Autodesk Fusion 360 part; units mm, degrees
sketch "Sketch1" plane through (0, 0, 0) normal (0, 1, 0) x (1, 0, 0)
  line L0 (-70, 0) -> (50, 0)
  line L1 (-70, 0) -> (-70, 20)
  line L2 (-70, 20) -> (-80, 20)
  line L3 (-80, 20) -> (-80, -20)
  line L4 (-80, -20) -> (50.3493, -2.6201)
  line L5 (50, 0) -> (50.3493, -2.6201)
  line L6 (-70.3109, -13.2) -> (-62.1109, -13.2)
  line L7 (-62.1109, -13.2) -> (-62.1109, -5)
  line L8 (-62.1109, -5) -> (-70.3109, -5)
  line L9 (-70.3109, -5) -> (-70.3109, -13.2)
  line L10 (-9.6566, -8.2) -> (-4.4566, -8.2)
  line L11 (-4.4566, -8.2) -> (-4.4566, -3)
  line L12 (-4.4566, -3) -> (-9.6566, -3)
  line L13 (-9.6566, -3) -> (-9.6566, -8.2)
  dimension "d1" = 20
  dimension "d2" = 10
  dimension "d3" = 40
  dimension "d4" = 8.2
  dimension "d5" = 8.2
  dimension "d6" = 5
  dimension "d7" = 5.2
  dimension "d8" = 5.2
  dimension "d9" = 3
extrude "Extrude1" add sketch "Sketch1" along normal blind 8
fillet "Fillet1" radius 2 1 edges at (-70, 4, 0)
fillet "Fillet2" radius 6 1 edges at (-80, 4, -20)
fillet "Fillet3" radius 2.5 1 edges at (-70, 4, -20)
fillet "Fillet4" radius 2.5 1 edges at (-80, 4, 20)
fillet "Fillet5" radius 1.2 2 edges at (50.3493, 4, 2.6201) (50, 4, 0)
The listing builds one solid part. Answer for the finished solid, in the listing's coordinates (mm). A direction names the side the tool comes from. Give positions to 0.01 mm unless a question says otherwise; leave off trailing zeros. Loops run counter-clockwise (first coordinate to the right, second up) from the corner with the lowest first, then second, coordinate; pieces in that order, holes last. Notation, with made-up numbers: (-20, -14.75) - (-12, -14.75) arc R31 ccw to (-12, 17.25) - close; hole circle Ø6 at (-8.5, 5). An arc over 180 degrees is marked (long way). Write each question's results on one line, items separated by ' | '.
1. Which of the six approach directions +Z, -Z, +X, -X, +Y, -Y give full straight-line access (tool end or side, diameter ignored) to faces 1 (the face through (-34, 8, 4)), 2 (the face through (-4.457, 4, 6))?
Resolved:
face 1: +Z, -Z, +X, -X, +Y | face 2: +Y, -Y
2. For a pull along X with two mould halves and no side action, classify faces 3 (the face through (-70, 4, -10)), 4 (the face through (-78.196, 4.056, -18.289)), 5 (the face through (-10, 4, 0)), 6 (the face through (-70.311, 4, 9)) as +X half, -X half, draft (parallel to the pull), parting line (faces both ways), or undercut.
Resolved:
face 3: +X half | face 4: -X half | face 5: draft | face 6: undercut
3. Flat-ended cylindrical pins translate along their axes: P1, Ø4, axis at x = -7.5, y = 5, coming from the +Z side; P2, Ø2.5, axis at x = -64.5, y = 4, coming from the +Z side; P3, Ø2.5, axis at y = 3, z = -7.5, coming from the +X side. Find the tip coordinate at first contact, or state that the pin passes through.
Resolved:
P1: stops at z = 10.6 | P2: stops at z = 18.1 | P3: stops at x = -70
4. Find section B-B, the plane x = 1. Write down the section's boundary in (y, z).
Resolved:
outline: (0, 0) - (8, 0) - (8, 9.2) - (0, 9.2) - close
5. Consider probe 1 along X at (y, z) = (7.5, 1); probe 2 along Z at (x, y) = (-66, 0.5); probe 3 along X at (y, z) = (6.5, -8.5). Determine where each line is inside the solid, lowest interval first. Write a range as from..to.
Resolved:
probe 1: x = -80..50.13 | probe 2: z = 0..5, 13.2..18.13 | probe 3: x = -80..-70
6. Find section A-A, the plane y = 3.75. Write down the section's boundary in (x, z), then the cut area to 3 significant figures.
Resolved:
outline: (-80, -14) arc R6 ccw to (-74, -20) - (-72.5, -20) arc R2.5 ccw to (-70, -17.5) - (-70, -2) arc R2 cw to (-68, 0) - (48.95, 0) arc R1.2 ccw to (50.14, 1.04) - (50.19, 1.43) arc R1.2 ccw to (49.16, 2.78) - (-77.17, 19.62) arc R2.5 ccw to (-80, 17.14) - close; hole (-70.31, 5) - (-62.11, 5) - (-62.11, 13.2) - (-70.31, 13.2) - close; hole (-9.66, 3) - (-4.46, 3) - (-4.46, 8.2) - (-9.66, 8.2) - close | area: 1,570 mm^2
7. Find section C-C, the plane z = -4.5. Write down the section's boundary in (x, y), then the cut area to 3 significant figures.
Resolved:
outline: (-80, 0) - (-70, 0) - (-70, 8) - (-80, 8) - close | area: 80.0 mm^2
